Answer from the drawing. Dimensions are ordinates in mm from the lowest x, y and z of the part. Coordinates: 2 decimals unless noted, no trailing zeros. Order: outer loops, then holes, each group sorted by start corner. A loop starts at its lowest first (then second) coordinate and runs counter-clockwise, first axis right, second up. Notation, with made-up numbers: (-18.5, 24.25) - (15.5, 24.25) arc R26 ccw to (15.5, 38.25) - close; hole circle Ø6 at (34.5, -29.5). An arc over 180 degrees is marked (long way). One line per item, written item: value. Start each with the question number.
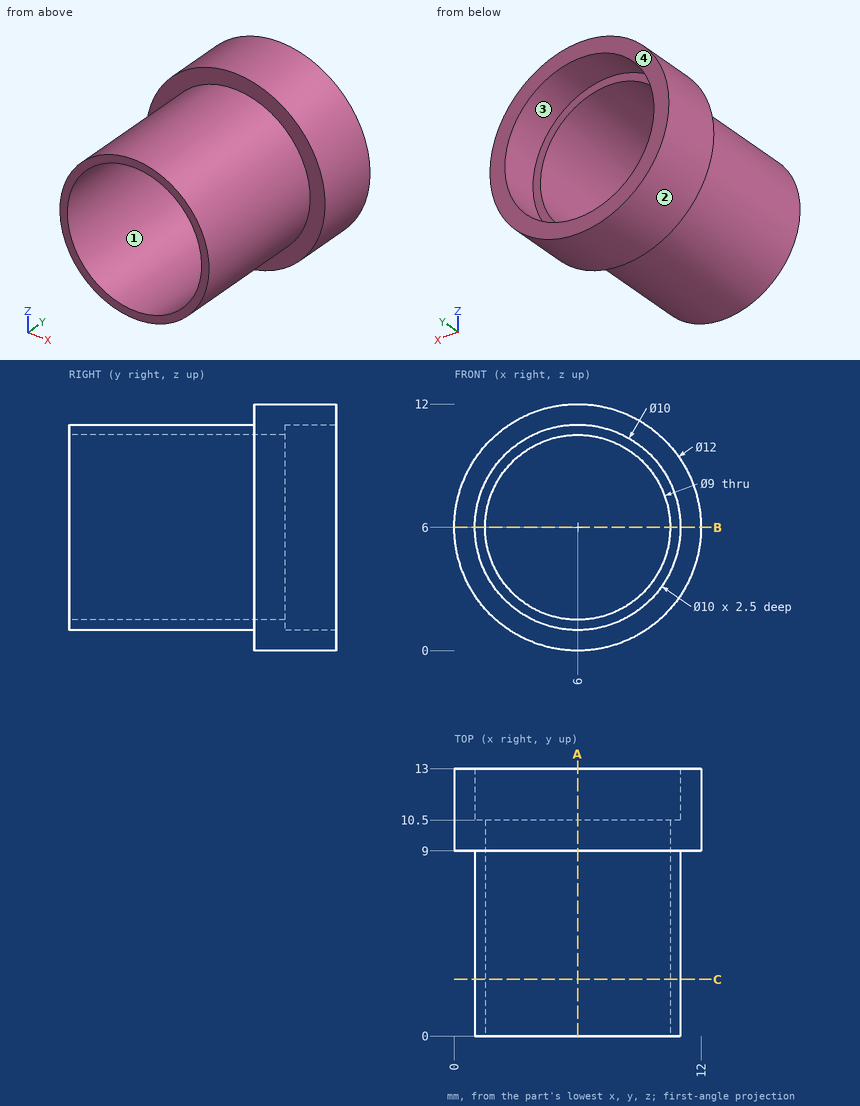
(1) The part is cut by section B-B on z = 6. Determine the outline of the cut face in (x, y), plus the area to 3 significant figures.
(2) Flat-ended cylindrical pins translate along their axes: pin 1 Ø4 at (y, z) = (4.5, 3.5) entering from +X; pin 2 Ø1.5 at (x, z) = (1.5, 5) entering from +Y; pin 3 Ø5 at (y, z) = (8.5, 3) entering from -X; pin 4 Ø4 at (y, z) = (2, 9.5) entering from +X. Find the tip coordinate at first contact, or state that the pin passes through.
(3) Consider probe 1 along X at (y, z) = (6.5, 6); probe 2 along X at (y, z) = (12.15, 6); probe 3 along Y at (x, z) = (9.75, 10.5). Determine where each line is inside the solid, lowest interval first.
(4) The part is cut by section A-A on x = 6. Determine the outline of the cut face in (y, z).
(5) The part is cut by section C-C on y = 2.75. Determine the outline of the cut face in (x, z), plus the area to 3 significant figures.
(6) For a pull along Z with two mould halves and no side action, classify the marked faces 1, 2, 3 and 4 as pulls with the +Z half, pulls with the -Z half, needs draft (parallel to the pull), parting line crosses it, or undercut.
Completed:
1. outline: (0, 9) - (1, 9) - (1, 0) - (1.5, 0) - (1.5, 10.5) - (1, 10.5) - (1, 13) - (0, 13) - close; (10.5, 0) - (11, 0) - (11, 9) - (12, 9) - (12, 13) - (11, 13) - (11, 10.5) - (10.5, 10.5) - close
1. area: 18.5 mm2
2. pin 1: stops at x = 10.97
2. pin 2: stops at y = 13
2. pin 3: stops at x = 0.03
2. pin 4: stops at x = 10.77
3. probe 1: x = 1 to 1.5, 10.5 to 11
3. probe 2: x = 0 to 1, 11 to 12
3. probe 3: y = 9 to 13
4. outline: (0, 1) - (9, 1) - (9, 0) - (13, 0) - (13, 1) - (10.5, 1) - (10.5, 1.5) - (0, 1.5) - close; (0, 10.5) - (10.5, 10.5) - (10.5, 11) - (13, 11) - (13, 12) - (9, 12) - (9, 11) - (0, 11) - close
5. outline: circle Ø10 at (6, 6); hole circle Ø9 at (6, 6)
5. area: 14.9 mm2
6. face 1: undercut
6. face 2: parting line crosses it
6. face 3: undercut
6. face 4: needs draft
